For this review, take the finished solid that the model builds, in its own axes (mm). Coordinates: 2 decimals unless noted, no trailing zeros. Write each loop counter-clockwise with the first axis right and the second up, starting at its lowest first coordinate (ties: lowest second). Pieces come first, ordered by that corner, then holes.
1) Insertion check: P1, Ø1, axis at y = -5, z = 8.5, coming from the -X side; P2, Ø6, axis at y = -0.5, z = 11.5, coming from the -X side; P3, Ø6, axis at x = 11, z = 4.5, coming from the +Y side; P4, Ø1.5, axis at x = 5.5, z = 10.5, coming from the -Y side. Each pin has a flat end and moves straight along its axis. Give the tip position at first contact, or say it passes through.
2) To check wall thickness, follow line 1 along Y through (x, z) = (7.5, 0); line 2 along Z through (x, y) = (7, 0); line 3 along Z through (x, y) = (11, 7.5). State the ranges of each line that lie inside material, in increasing order.
3) We need section A-A on x = 5. Write out the cut boundary in (y, z).
4) Mouldability with a two-part tool opening along Z and no side actions: class faces 1 (the face through (6.4, -13.8, 8.1)), 2 (the face through (0.347, -16.602, -0.041)), 3 (the face through (6.58, 9.718, -3.06)) as pulls with the +Z half, pulls with the -Z half, needs draft (parallel to the pull), parting line crosses it, or undercut.
from build123d import *

# Parameters (mm, degrees)
SKETCH_2_W          = 64
SKETCH_2_H          = 64
CUT_EXTRUDE_1_DEPTH = 26


with BuildPart() as part:
    # 草图1 → 旋转1 (revolve)
    with BuildSketch(Plane.XY):
        Polygon((0, 0), (0, 16), (1.847520861, 19.2), (11.152479139, 19.2), (13, 16), (13, 0), align=None)
    revolve(axis=Axis((13, 0, 0), (-1, 0, 0)))

    # 草图2 → 切除-拉伸1 (cut)
    with BuildSketch(Plane(origin=(0, 0, 0), x_dir=(0, 0, -1), z_dir=(1, 0, 0))):
        Rectangle(SKETCH_2_W, SKETCH_2_H)
        Polygon((-16, -9.237604307), (0, -18.475208614), (16, -9.237604307), (16, 9.237604307), (0, 18.475208614), (-16, 9.237604307), align=None, mode=Mode.SUBTRACT)
    extrude(amount=CUT_EXTRUDE_1_DEPTH, mode=Mode.SUBTRACT)

    # 草图3 → 切除-旋转1 (revolve, cut)
    with BuildSketch(Plane.XY):
        Polygon((0, 0), (0, 11), (0.812, 10.188), (12.188, 10.188), (13, 11), (13, 0), align=None)
    revolve(axis=Axis((13, 0, 0), (-1, 0, 0)), mode=Mode.SUBTRACT)


solid = part.part
Result:
1. P1: stops at x = 0.64
1. P2: stops at x = 0
1. P3: stops at y = 17.61
1. P4: stops at y = -12.85
2. line 1: y = -18.48 to -10.19, 10.19 to 18.48
2. line 2: z = -16 to -10.19, 10.19 to 16
2. line 3: z = -16 to -6.9, 6.9 to 16
3. outline: (-18.48, 0) - (-9.24, -16) - (9.24, -16) - (18.48, 0) - (9.24, 16) - (-9.24, 16) - close; hole circle Ø20.38 at (0, 0)
4. face 1: pulls with the +Z half
4. face 2: parting line crosses it
4. face 3: undercut
